CAD build for the part. Positions are in the model's coordinates, mm. A direction names the side the tool comes from. Coordinates: 2 decimals unless noted, no trailing zeros. Loops run counter-clockwise (first coordinate to the right, second up) from the corner with the lowest first, then second, coordinate; pieces in that order, holes last. Notation, with made-up numbers: (-30, -27) -> (-20, -27) arc R4 ccw to (-20, -20) -> close; hole circle Ø8 at (63, 35.25). An arc over 180 degrees is marked (long way). Write each question's results on one line, items separated by ' | '.
```python
from build123d import *

# Parameters (mm, degrees)
F1_DEPTH = 20
F2_DEPTH = 25
F3_R     = 1


with BuildPart() as f1:
    # F0 (on Front) → F1 (new body)
    with BuildSketch(Plane.XZ):
        with BuildLine():
            Line((25, 27), (-25, 27))
            ThreePointArc((-25, 27), (-40.556349, 20.556349), (-47, 5))
            Line((-47, 5), (-47, -5))
            ThreePointArc((-47, -5), (-36.162951, -31.162951), (-10, -42))
            Line((-10, -42), (10, -42))
            ThreePointArc((10, -42), (36.162951, -31.162951), (47, -5))
            Line((47, -5), (47, 5))
            ThreePointArc((47, 5), (40.556349, 20.556349), (25, 27))
        make_face()
    extrude(amount=F1_DEPTH)

    # F0 (on Front) → F2 (join)
    with BuildSketch(Plane.XZ):
        with BuildLine():
            ThreePointArc((10, -45), (38.284271, -33.284271), (50, -5))
            Line((50, -5), (50, 5))
            ThreePointArc((50, 5), (42.67767, 22.67767), (25, 30))
            Line((25, 30), (-25, 30))
            ThreePointArc((-25, 30), (-42.67767, 22.67767), (-50, 5))
            Line((-50, 5), (-50, -5))
            ThreePointArc((-50, -5), (-38.284271, -33.284271), (-10, -45))
            Line((-10, -45), (10, -45))
        make_face()
        with BuildLine():
            ThreePointArc((-47, 5), (-40.556349, 20.556349), (-25, 27))
            Line((-25, 27), (25, 27))
            ThreePointArc((25, 27), (40.556349, 20.556349), (47, 5))
            Line((47, 5), (47, -5))
            ThreePointArc((47, -5), (36.162951, -31.162951), (10, -42))
            Line((10, -42), (-10, -42))
            ThreePointArc((-10, -42), (-36.162951, -31.162951), (-47, -5))
            Line((-47, -5), (-47, 5))
        make_face(mode=Mode.SUBTRACT)
    extrude(amount=F2_DEPTH)

    # F3
    f3_edges = [f1.edges().sort_by_distance(p)[0] for p in [
        (0, -25, 27),
        (38.284271, -25, -33.284271),
    ]]
    fillet(f3_edges, radius=F3_R)


solid = f1.part
```
Q1. Pull direction Z, two halves, no side cores. Call faces 1 (the flat face through (0, -12, -45)), 2 (the cylindrical face through (-42.482, -11.832, 22.871)), 3 (the flat face through (50, -12, 0)), 4 (the cylindrical face through (-35.87, -21.97, -31.45)): +Z half, -Z half, draft (parallel to the pull), parting line (faces both ways), or undercut.
Results are:
face 1: -Z half | face 2: +Z half | face 3: draft | face 4: undercut
Q2. Cut at A-A on y = -22. Write the cut outline in (x, z).
Results are:
outline: (-50, -5) arc R40 ccw to (-10, -45) -> (10, -45) arc R40 ccw to (50, -5) -> (50, 5) arc R25 ccw to (25, 30) -> (-25, 30) arc R25 ccw to (-50, 5) -> close; hole (-47, -5) arc R37 ccw to (-10, -42) -> (10, -42) arc R37 ccw to (47, -5) -> (47, 5) arc R22 ccw to (25, 27) -> (-25, 27) arc R22 ccw to (-47, 5) -> close
Q3. Cut at B-B on z = -3. Write the cut outline in (x, y).
Results are:
outline: (-50, -24) arc R1 ccw to (-49, -25) -> (-48, -25) arc R1 ccw to (-47, -24) -> (-47, -20) -> (47, -20) -> (47, -24) arc R1 ccw to (48, -25) -> (49, -25) arc R1 ccw to (50, -24) -> (50, 0) -> (-50, 0) -> close
Q4. Which spindle directions (+Z, -Z, +X, -X, +Y, -Y) get a long thin tool onto all of the face, cutting with end or side? Do faces 5 (the flat face through (47, -22, 0)), 6 (the cylindrical face through (37.972, -11.832, -33.594)). Say none if no direction does.
Results are:
face 5: -Y | face 6: -Z, +X, +Y, -Y
Q5. Drop flat-ended pins along their axis: pin 1 (4 mm diameter, centred on x = -11.5, z = 1, fed in from -Y); pin 2 (5 mm diameter, centred on y = -20, z = -14, fed in from +X); pin 3 (10 mm diameter, centred on y = -5.5, z = 12.5, fed in from -X). Give the stop position or say it passes through.
Results are:
pin 1: y = -20 | pin 2: x = 49.47 | pin 3: x = -49.87
Q6. Cut at C-C on y = -15.5. Write the cut outline in (x, z), and give its area (3 significant figures).
Results are:
outline: (-50, -5) arc R40 ccw to (-10, -45) -> (10, -45) arc R40 ccw to (50, -5) -> (50, 5) arc R25 ccw to (25, 30) -> (-25, 30) arc R25 ccw to (-50, 5) -> close | area: 6,550 mm^2
Q7. Wall check: L1, parallel to X at y = -23.5, z = -5.5; L2, parallel to Y at x = 25, z = -31.5; L3, parallel to Z at x = 42, y = -20.5. Give the ranges that are in metal, low to high. Write a range as from..to.
Results are:
L1: -50..-47, 47..50 | L2: -20..0 | L3: -29..-23.57, 18.96..23.33
